Autodesk Inventor part; units mm, degrees
ref_plane "YZ Plane" through (0, 0, 0) normal (1, 0, 0) x (0, 1, 0)
ref_plane "XZ Plane" through (0, 0, 0) normal (0, 1, 0) x (-1, 0, 0)
ref_plane "XY Plane" through (0, 0, 0) normal (0, 0, 1) x (1, 0, 0)
sketch "Sketch1" plane through (0, 0, 0) normal (0, 1, 0) x (-1, 0, 0)
  line L0 (0, 0) -> (63.5, 0)
  line L1 (63.5, 0) -> (63.5, -36.068)
  line L2 (63.5, -36.068) -> (0, -36.068)
  line L3 (0, -36.068) -> (0, 0)
  dimension "d0" = 63.5
  dimension "d1" = 36.068
extrude "Extrusion1" add sketch "Sketch1" along normal blind 3.81
sketch "Sketch2" plane through (0, 0, 0) normal (1, 0, 0) x (0, 0, -1)
  point P0 (0, 0)
fillet "Fillet1" radius 1.27 12 edges at (-31.75, 3.81, 0) (-31.75, 3.81, -36.068) (-31.75, 0, 0) (-31.75, 0, -36.068) (0, 0, -18.034) (0, 3.81, -18.034) (0, 1.905, 0) (0, 1.905, -36.068) (-63.5, 1.905, -36.068) (-63.5, 3.81, -18.034) (-63.5, 1.905, 0) (-63.5, 0, -18.034)
properties part number "battery"
Can you work these out from the model? Positions are in its coordinate system, mm. Round coordinates to 2 decimals unless told otherwise and drop trailing zeros. Loops run counter-clockwise (first coordinate to the right, second up) from the corner with the lowest first, then second, coordinate; pieces in that order, holes last. Notation, with made-up numbers: (69.5, 56) -> (76.5, 56) arc R30 ccw to (76.5, 82) -> close; hole circle Ø11 at (26, -1.5). An arc over 180 degrees is marked (long way). Answer in a Markdown table with one row per item.
Item 1: Suppose I cut it at A-A, the plane y = 0.6. List the corners of the cut face in (x, z) for me.
Answer block:
| item | result |
|---|---|
| outline | (-63.31, -34.8) arc R1.08 ccw to (-62.23, -35.88) -> (-1.27, -35.88) arc R1.08 ccw to (-0.19, -34.8) -> (-0.19, -1.27) arc R1.08 ccw to (-1.27, -0.19) -> (-62.23, -0.19) arc R1.08 ccw to (-63.31, -1.27) -> close |
Item 2: If I drill on probe 1 along Z at (x, y) = (-15.5, 1.15); probe 2 along Z at (x, y) = (-31.5, 2.95); probe 3 along X at (y, z) = (0.45, -4), over which ranges is the centre line in solid material (lowest first)?
Answer block:
| item | result |
|---|---|
| probe 1 | -36.06 to -0.01 |
| probe 2 | -36 to -0.07 |
| probe 3 | -63.2 to -0.3 |
Item 3: Will this pin go through, and if not, where does the flat tip stop? P1, Ø1, axis at x = -24.5, z = -22, coming from the -Y side.
Answer block:
| item | result |
|---|---|
| P1 | y = 0 |
